For this review, take the finished solid that the model builds, in its own axes (mm). A direction names the side the tool comes from. Coordinates: 2 decimals unless noted, no trailing zeros. Write each loop counter-clockwise with the first axis right and the second up, starting at its lowest first coordinate (ties: lowest second). Pieces come first, ordered by that corner, then holes. Notation, with made-up numbers: M -10,83 L 3,83 A25 cw 3,104 Z; hole C -11,-10 d5. An arc over 180 degrees is marked long. One line per question, with ' | ' between items.
from build123d import *

# Parameters (mm, degrees)
BOSS_EXTRUDE1_DEPTH      = 50
BOSS_EXTRUDE1_DEPTH_BACK = 50
CUT_EXTRUDE1_DEPTH       = 50
CUT_EXTRUDE1_DEPTH_BACK  = 50
SKETCH2_R                = 6.35


with BuildPart() as part:
    # Sketch1 → Boss-Extrude1 (new, two sides: drawn at the far end of the back side and taken through both)
    with BuildSketch(Plane(origin=(0, 0, 0), x_dir=(0, 0, -1), z_dir=(1, 0, 0)).offset(-BOSS_EXTRUDE1_DEPTH_BACK)):
        Polygon((0, 0), (0, 100), (-6.35, 100), (-6.35, -6.35), (100, -6.35), (100, 0), align=None)
    extrude(amount=BOSS_EXTRUDE1_DEPTH + BOSS_EXTRUDE1_DEPTH_BACK)

    # Sketch2 → Cut-Extrude1 (cut, two sides: drawn at the far end of the back side and taken through both)
    with BuildSketch(Plane.XY.offset(-CUT_EXTRUDE1_DEPTH_BACK)):
        with Locations(Location((0, 50, 0), (0, 0, 180))):
            Circle(SKETCH2_R)
    extrude(amount=CUT_EXTRUDE1_DEPTH + CUT_EXTRUDE1_DEPTH_BACK, mode=Mode.SUBTRACT)


solid = part.part
1) We need section D-D on z = -79. State the section outline as (x, y) points.
Responses:
outline: M -50,-6.35 L 50,-6.35 L 50,0 L -50,0 Z
2) To check wall thickness, follow line 1 along Z through (x, y) = (28, 29.5); line 2 along Y through (x, z) = (9.5, -34.5); line 3 along Y through (x, z) = (0, 4.5). State the ranges of each line that lie inside material, in increasing order. Write a range as [from, to].
Responses:
line 1: [0, 6.35] | line 2: [-6.35, 0] | line 3: [-6.35, 43.65], [56.35, 100]
3) We need section A-A on y = 50. State the section outline as (x, z) points, then the cut area to 3 significant figures.
Responses:
outline: M -50,0 L -6.35,0 L -6.35,6.35 L -50,6.35 Z; M 6.35,0 L 50,0 L 50,6.35 L 6.35,6.35 Z | area: 554 mm^2
4) The part is to be moulded in two halves that separate along X. For faces 3 (the flat face through (-50, 23, 1)), 4 (the flat face through (-1, 100, 3)), 5 (the flat face through (50, 23, 1)), 6 (the cylindrical face through (1.38, 56.2, 3.13)), say which applies: +X half, -X half, draft (parallel to the pull), parting line (faces both ways), or undercut.
Responses:
face 3: -X half | face 4: draft | face 5: +X half | face 6: undercut
5) We need section B-B on x = 0. State the section outline as (y, z) points, then the cut area to 3 significant figures.
Responses:
outline: M -6.35,-100 L 0,-100 L 0,0 L 43.65,0 L 43.65,6.35 L -6.35,6.35 Z; M 56.35,0 L 100,0 L 100,6.35 L 56.35,6.35 Z | area: 1,230 mm^2
6) Machinability: for faces 1 (the flat face through (-1, 38, 0)), 2 (the flat face through (-12, 48, 6.35)), which of the approach directions +Z, -Z, +X, -X, +Y, -Y give a long, thin tool a straight path to every point of the face, cutting with its end or side? Answer none if there is none.
Responses:
face 1: -Z, +X, -X, +Y | face 2: +Z, +X, -X, +Y, -Y
7) We need section C-C on x = 37.5. State the section outline as (y, z) points, then the cut area to 3 significant figures.
Responses:
outline: M -6.35,-100 L 0,-100 L 0,0 L 100,0 L 100,6.35 L -6.35,6.35 Z | area: 1,310 mm^2
8) Insertion check: pin 1 Ø10 at (x, y) = (-13.5, 88) entering from -Z; pin 2 Ø5 at (x, z) = (17, -21) entering from +Y. Each pin has a flat end and moves straight along its axis. Give the tip position at first contact, or say it passes through.
Responses:
pin 1: z = 0 | pin 2: y = 0
